from build123d import *
from build123d.topology import SkipClean

# Parameters (mm, degrees)
CROQUIS1_R              = 47.5
CROQUIS1_R_2            = 3.175
CROQUIS1_R_3            = 15
SALIENTE_EXTRUIR1_DEPTH = 7
SALIENTE_EXTRUIR2_START = 48
CROQUIS2_R              = 19
CROQUIS2_R_2            = 15
SALIENTE_EXTRUIR2_DEPTH = 48
SALIENTE_EXTRUIR3_START = 3
CROQUIS3_R              = 7.5
CROQUIS3_R_2            = 3.175
SALIENTE_EXTRUIR3_DEPTH = 3


with BuildPart() as part:
    # Croquis1 → Saliente-Extruir1 (new body)
    with BuildSketch(Plane(origin=(0, 0, 0), x_dir=(1, 0, 0), z_dir=(0, 1, 0))):
        with Locations(Location((0, 0, 0), (0, 0, 270))):
            Circle(CROQUIS1_R)
        with Locations(Location((0, 32, 0), (0, 0, 270))):
            Circle(CROQUIS1_R_2, mode=Mode.SUBTRACT)
        with Locations(Location((27.712812921, -16, 0), (0, 0, 270))):
            Circle(CROQUIS1_R_2, mode=Mode.SUBTRACT)
        with Locations(Location((-27.712812921, -16, 0), (0, 0, 270))):
            Circle(CROQUIS1_R_2, mode=Mode.SUBTRACT)
        with Locations(Location((0, 0, 0), (0, 0, 270))):
            Circle(CROQUIS1_R_3, mode=Mode.SUBTRACT)
    extrude(amount=SALIENTE_EXTRUIR1_DEPTH)

    # Croquis2 → Saliente-Extruir2 (add)
    with SkipClean():  # the faces are left unmerged after this step: merging them gives an invalid solid
        with BuildSketch(Plane.XZ.offset(SALIENTE_EXTRUIR2_START)):
            with Locations(Location((0, 0, 0), (0, 0, 90))):
                Circle(CROQUIS2_R)
            with Locations(Location((0, 0, 0), (0, 0, 270))):
                Circle(CROQUIS2_R_2, mode=Mode.SUBTRACT)
        extrude(amount=-SALIENTE_EXTRUIR2_DEPTH)

    # Croquis3 → Saliente-Extruir3 (add)
    # profile 1 of 3: a face of its own
    with SkipClean():  # the faces are left unmerged after this step: merging them gives an invalid solid
        with BuildSketch(Plane.XZ.offset(SALIENTE_EXTRUIR3_START)):
            with Locations(Location((-27.712812921, 16, 0), (0, 0, 90))):
                Circle(CROQUIS3_R)
            with Locations(Location((-27.712812921, 16, 0), (0, 0, 270))):
                Circle(CROQUIS3_R_2, mode=Mode.SUBTRACT)
        # profile 2 of 3: a face of its own
        with BuildSketch(Plane.XZ.offset(SALIENTE_EXTRUIR3_START)):
            with Locations(Location((27.712812921, 16, 0), (0, 0, 90))):
                Circle(CROQUIS3_R)
            with Locations(Location((27.712812921, 16, 0), (0, 0, 270))):
                Circle(CROQUIS3_R_2, mode=Mode.SUBTRACT)
        # profile 3 of 3: a face of its own
        with BuildSketch(Plane.XZ.offset(SALIENTE_EXTRUIR3_START)):
            with Locations(Location((0, -32, 0), (0, 0, 90))):
                Circle(CROQUIS3_R)
            with Locations(Location((0, -32, 0), (0, 0, 270))):
                Circle(CROQUIS3_R_2, mode=Mode.SUBTRACT)
        extrude(amount=-SALIENTE_EXTRUIR3_DEPTH)


solid = part.part
Read the model definition and answer for the solid it produces. Units are mm, in the model's axes. A direction names the side the tool comes from. Round coordinates to 2 decimals unless told otherwise and drop trailing zeros. Order: outer loops, then holes, each group sorted by start corner. A loop starts at its lowest first (then second) coordinate and runs counter-clockwise, first axis right, second up.
1) Flat-ended cylindrical pins translate along their axes: pin 1 (1 mm diameter, centred on x = -7.5, y = -6.5, fed in from -Z); pin 2 (8 mm diameter, centred on x = -26.5, y = -35, fed in from +Z); pin 3 (1 mm diameter, centred on y = -10.5, z = -11.5, fed in from +X); pin 4 (7.5 mm diameter, centred on x = 1.5, z = -34, fed in from -Y). Find the tip coordinate at first contact, or state that the pin passes through.
2) Straight lines are drawn through the part: L1, parallel to X at y = -25, z = 0; L2, parallel to X at y = -2.2, z = -32 (3 decimals); L3, parallel to X at y = 4, z = 16. For each, find the intervals that lie inside material, in ascending order.
3) The mould has two halves that part along X. Classify faces 5 (the face through (20.277, -1.521, 15.024)), 6 (the face through (-0.33, -1.521, -39.493)), 7 (the face through (29.3, -3, 19.2)): released by +X, released by -X, zero draft, split by the parting line, or undercut.
4) The part is cut by section C-C on x = 10. Write down the section's boundary in (y, z), plus the area to 3 significant figures.
5) The part is cut by section D-D on y = -43. Write down the section's boundary in (x, z), plus the area to 3 significant figures.
6) The part is cut by section B-B on x = 0. Write down the section's boundary in (y, z) (3 decimals), plus the area to 4 significant figures.
7) The part is cut by section A-A on z = 0. Write down the section's boundary in (x, y), plus the area to 3 significant figures.
8) For faces 1 (the face through (3, -3, -30)), 2 (the face through (-24, -3, 16)), 3 (the face through (-20, 0, -1)), 4 (the face through (11, 7, -11)), determine the directions among +Z, -Z, +X, -X, +Y, -Y from which every point of the face is accessible in a straight line to the end or side of a thin tool.
Resolved:
1. pin 1: stops at z = -17.66
1. pin 2: passes through
1. pin 3: stops at x = 15.49
1. pin 4: stops at y = -3
2. L1: x = -19 to -15, 15 to 19
2. L2: x = -7.5 to -3.175, 3.175 to 7.5
2. L3: x = -44.72 to -30.89, -24.54 to 24.54, 30.89 to 44.72
3. face 5: undercut
3. face 6: split by the parting line
3. face 7: zero draft
4. outline: (-48, -16.16) - (0, -16.16) - (0, -46.44) - (7, -46.44) - (7, -11.18) - (-48, -11.18) - close; (-48, 11.18) - (7, 11.18) - (7, 46.44) - (0, 46.44) - (0, 16.16) - (-48, 16.16) - close
4. area: 971 mm2
5. outline: circle Ø38 at (0, 0); hole circle Ø30 at (0, 0)
5. area: 427 mm2
6. outline: (-48, -19) - (0, -19) - (0, -24.5) - (-3, -24.5) - (-3, -28.825) - (7, -28.825) - (7, -15) - (-48, -15) - close; (-48, 15) - (7, 15) - (7, 47.5) - (0, 47.5) - (0, 19) - (-48, 19) - close; (-3, -39.5) - (0, -39.5) - (0, -47.5) - (7, -47.5) - (7, -35.175) - (-3, -35.175) - close
6. area: 820.5 mm2
7. outline: (-47.5, 0) - (-19, 0) - (-19, -48) - (-15, -48) - (-15, 7) - (-47.5, 7) - close; (15, -48) - (19, -48) - (19, 0) - (47.5, 0) - (47.5, 7) - (15, 7) - close
7. area: 839 mm2
8. face 1: -Z, +X, -X, -Y
8. face 2: +Z, -Z, -X, -Y
8. face 3: -Y
8. face 4: +Z, -Z, +X, -X, +Y
